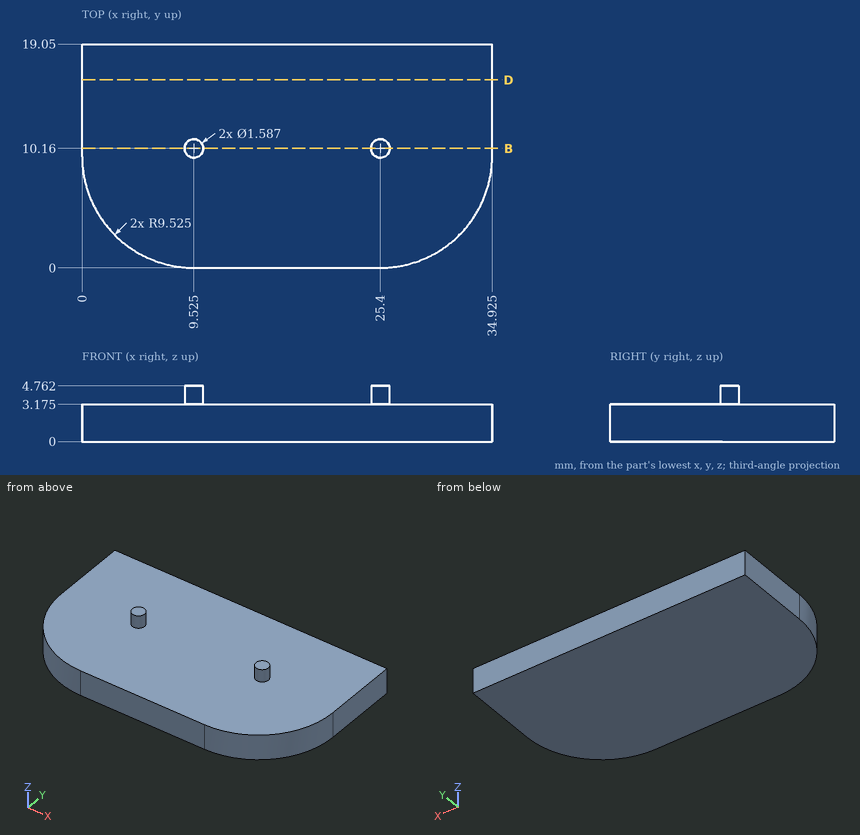
Verification items for this drawing (mm, ordinates from the low corner). Round coordinates to 2 decimals unless told otherwise and drop trailing zeros. Loops run counter-clockwise (first coordinate to the right, second up) from the corner with the lowest first, then second, coordinate; pieces in that order, holes last. Notation, with made-up numbers: (3.25, -15) -> (46.25, -15) arc R27 cw to (46.25, 17) -> close; hole circle Ø6 at (16, 10.5). An arc over 180 degrees is marked (long way). Answer in a Markdown table with one row per item.
Q1. Sectioned sample at B-B on y = 10.16. Enter the section's corners in (x, z) (1 decimal), then the cut area to 3 significant figures.
Data:
| item | result |
|---|---|
| outline | (0, 0) -> (34.9, 0) -> (34.9, 3.2) -> (26.2, 3.2) -> (26.2, 4.8) -> (24.6, 4.8) -> (24.6, 3.2) -> (10.3, 3.2) -> (10.3, 4.8) -> (8.7, 4.8) -> (8.7, 3.2) -> (0, 3.2) -> close |
| area | 116 mm^2 |
Q2. Thickness scan on L1, parallel to Z at x = 16, y = 7.5 (1 decimal); L2, parallel to X at y = 10, z = 4; L3, parallel to Y at x = 31, z = 1.15. Record the ranges inside material, lowest first.
Data:
| item | result |
|---|---|
| L1 | z = 0 to 3.2 |
| L2 | x = 8.75 to 10.3, 24.62 to 26.18 |
| L3 | y = 1.82 to 19.05 |
Q3. Sectioned sample at D-D on y = 16. Enter the section's corners in (x, z) (1 decimal), then the cut area to 3 significant figures.
Data:
| item | result |
|---|---|
| outline | (0, 0) -> (34.9, 0) -> (34.9, 3.2) -> (0, 3.2) -> close |
| area | 111 mm^2 |
Q4. Go/stop test with a flat-tipped pin: P1, Ø5.5, axis at x = 17, y = 8.5, coming from the +Z side (1 decimal). Record where the tip stops, or that it passes through.
Data:
| item | result |
|---|---|
| P1 | stops at z = 3.2 |
